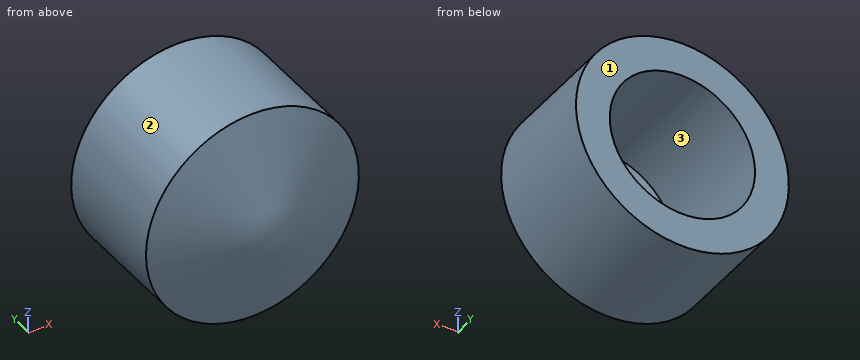
from build123d import *
from OCP.BRepAlgoAPI import BRepAlgoAPI_Cut
from OCP.TopTools import TopTools_ListOfShape

# Parameters (mm, degrees)
SKETCH1_R           = 8.001
SKETCH1_R_2         = 5.461
BOSS_EXTRUDE1_DEPTH = 8.864442387
CUT_EXTRUDE1_START  = 8.864442
SKETCH1_6_R         = 5.461
CUT_EXTRUDE1_DEPTH  = 9.46


with BuildPart() as part:
    # Sketch1 → Boss-Extrude1 (new body)
    # profile 1 of 2: a face of its own
    with BuildSketch(Plane(origin=(0, 0, 0), x_dir=(1, 0, 0), z_dir=(0, 1, 0))):
        with Locations(Location((0, 0, 0), (0, 0, 270))):
            Circle(SKETCH1_R)
        Circle(SKETCH1_R_2, mode=Mode.SUBTRACT)
    # profile 2 of 2: a face of its own
    with BuildSketch(Plane(origin=(0, 0, 0), x_dir=(1, 0, 0), z_dir=(0, 1, 0))):
        Circle(SKETCH1_R_2)
    extrude(amount=BOSS_EXTRUDE1_DEPTH)

    # Sketch2 → Revolve1 (revolve)
    with BuildSketch(Plane.XY, mode=Mode.PRIVATE) as revolve1_sk:
        Polygon((0, 0), (0, -3.135557613), (8.001, 0), align=None)
    revolve(revolve1_sk.sketch.rotate(Axis((0, 0, 0), (0, -1, 0)), 180), axis=Axis((0, 0, 0), (0, -1, 0)))


with BuildPart() as cut_extrude1_tool:
    # Sketch1<6> → Cut-Extrude1 (new body)
    with BuildSketch(Plane(origin=(0, 0, 0), x_dir=(1, 0, 0), z_dir=(0, 1, 0)).offset(CUT_EXTRUDE1_START)):
        with Locations(Location((0, 0, 0), (0, 0, 270))):
            Circle(SKETCH1_6_R)
    extrude(amount=-CUT_EXTRUDE1_DEPTH)


with BuildPart() as part_1:
    add(part.part)

    # Cut-Extrude1: cut by cut_extrude1_tool, with a tolerance
    cut_extrude1_stock = TopTools_ListOfShape()
    cut_extrude1_stock.Append(part_1.part.wrapped)
    cut_extrude1_tools = TopTools_ListOfShape()
    cut_extrude1_tools.Append(cut_extrude1_tool.part.wrapped)
    cut_extrude1_cut = BRepAlgoAPI_Cut()
    cut_extrude1_cut.SetArguments(cut_extrude1_stock)
    cut_extrude1_cut.SetTools(cut_extrude1_tools)
    cut_extrude1_cut.SetFuzzyValue(0.00001)
    cut_extrude1_cut.Build()
    add(Compound.cast(cut_extrude1_cut.Shape()).solids(), mode=Mode.REPLACE)


solid = part_1.part
Geometry check sheet. Reference: the model listing, model coordinates, mm. Face numbers are marked on the shaded views. Give positions to 0.01 mm unless a question says otherwise; leave off trailing zeros. Loops run counter-clockwise (first coordinate to the right, second up) from the corner with the lowest first, then second, coordinate; pieces in that order, holes last.
(1) Section check B-B on y = -2. Record the cut outline in (x, z).
From the geometry:
outline: circle Ø5.8 at (0, 0)
(2) Depth check by flat-ended pin: pin 1 Ø3 at (x, y) = (6, 5.5) entering from +Z; pin 2 Ø2 at (x, y) = (5, 6) entering from -Z; pin 3 Ø4 at (y, z) = (-0.5, 4) entering from +X. Enter the tip coordinate at first touch or a pass-through.
From the geometry:
pin 1: stops at z = 6.62
pin 2: stops at z = -6.93
pin 3: stops at x = 7.73
(3) Thickness scan on L1, parallel to X at y = 6.25, z = 0; L2, parallel to Z at x = 4.25, y = 7.25; L3, parallel to X at y = 3, z = -4.5. Record the ranges inside material, lowest first.
From the geometry:
L1: x = -8 to -5.46, 5.46 to 8
L2: z = -6.78 to -3.43, 3.43 to 6.78
L3: x = -6.62 to -3.09, 3.09 to 6.62
(4) Section check A-A on y = 5.5. Record the cut outline in (x, z), then the cut area to 3 significant figures.
From the geometry:
outline: circle Ø16 at (0, 0); hole circle Ø10.92 at (0, 0)
area: 107 mm2
(5) Release check for a two-part mould opening along Z. For the marked faces 1, 2 and 3 record: released by +Z, released by -Z, zero draft, split by the parting line, or undercut.
From the geometry:
face 1: zero draft
face 2: split by the parting line
face 3: undercut
